Design review of the part built by this model. Coordinates are the model's own, in mm. A direction names the side the tool comes from. Round coordinates to 2 decimals unless told otherwise and drop trailing zeros. Loops run counter-clockwise (first coordinate to the right, second up) from the corner with the lowest first, then second, coordinate; pieces in that order, holes last. Notation, with made-up numbers: (25.5, 57.25) -> (55.5, 57.25) arc R25 ccw to (55.5, 75.25) -> close; hole circle Ø5 at (62, -26). An arc over 180 degrees is marked (long way). Write each question's results on one line, items separated by ' | '. Start each with the question number.
from build123d import *

# Parameters (mm, degrees)
F0_W      = 113
F0_H      = 75
F1_DEPTH  = 0.6
F2_W      = 113
F2_H      = 15
F3_DEPTH  = 1.8
F5_W      = 30
F5_H      = 8
F6_DEPTH  = 39
F8_DEPTH  = 3.4
F10_DEPTH = 4
F12_DEPTH = 2.4
F14_DEPTH = 28
F15_W     = 4
F15_H     = 2
F16_DEPTH = 5.4
F18_DEPTH = 9
F19_R     = 3
F22_DEPTH = 13
F24_DEPTH = 4
F25_R     = 1.6
F26_DEPTH = 2.4
F28_DEPTH = 1
F29_W     = 3
F29_H     = 2.8
F30_DEPTH = 5.6
F31_W     = 6
F31_H     = 3
F32_DEPTH = 3
F33_W     = 6
F33_H     = 3
F34_DEPTH = 6
F35_R     = 2
F36_DEPTH = 4


with BuildPart() as f1:
    # F0 (on Top) → F1 (new body)
    with BuildSketch(Plane.XY):
        with Locations((0, 37.5)):
            Rectangle(F0_W, F0_H)
    extrude(amount=F1_DEPTH)

    # F2 (on face) → F3 (join)
    with BuildSketch(Plane.XY.offset(0.6)):
        with Locations((0, 67.5)):
            Rectangle(F2_W, F2_H)
    extrude(amount=F3_DEPTH)

    # F5 (on offset) → F6 (join)
    with BuildSketch(Plane.YZ.offset(10)):
        with Locations((21, 4.6)):
            Rectangle(F5_W, F5_H)
    extrude(amount=F6_DEPTH)

    # F7 (on face) → F8 (join)
    with BuildSketch(Plane.XY.offset(0.6)):
        Polygon((-26, 17), (-54, 17), (-54, 8), (10, 8), (10, 39), (-26, 39), align=None)
    extrude(amount=F8_DEPTH)

    # F9 (on face) → F10 (join)
    with BuildSketch(Plane.XY.offset(4)):
        Polygon((-26, 26.13884), (-26, 17), (1.574617, 21.862149), (0.011783, 30.725419), align=None)
    extrude(amount=F10_DEPTH)

    # F11 (on face) → F12 (join)
    with BuildSketch(Plane.XY.offset(0.6)):
        with BuildLine():
            Line((-26, 39), (-19, 39))
            Line((-19, 39), (-22.779166, 43.858928))
            ThreePointArc((-22.779166, 43.858928), (-24.784166, 44.456406), (-26, 42.753835))
            Line((-26, 42.753835), (-26, 39))
        make_face()
    extrude(amount=F12_DEPTH)

    # F13 (on face) → F14 (join)
    with BuildSketch(Plane(origin=(-26, 0, 0), x_dir=(0, -1, 0), z_dir=(-1, 0, 0))):
        with BuildLine():
            ThreePointArc((-26.552914, 6.395555), (-30.374719, 4.530004), (-32, 0.6))
            Line((-32, 0.6), (-25, 0.6))
            Line((-25, 0.6), (-26.552914, 6.395555))
        make_face()
    extrude(amount=F14_DEPTH)

    # F15 (on face) → F16 (join)
    with BuildSketch(Plane.XY.offset(0.6)):
        with Locations((-45, 29.4)):
            Rectangle(F15_W, F15_H)
        with Locations((-36, 29.4)):
            Rectangle(F15_W, F15_H)
    extrude(amount=F16_DEPTH)

    # F17 (on face) → F18 (join)
    with BuildSketch(Plane.XY.offset(0.6)):
        with BuildLine():
            Line((18.5, 45.616959), (29.971529, 62))
            ThreePointArc((29.971529, 62), (18.5, 65.616959), (7.028471, 62))
            Line((7.028471, 62), (18.5, 45.616959))
        make_face()
    extrude(amount=F18_DEPTH)

    # F19
    f19_edges = [f1.edges().sort_by_distance(p)[0] for p in [
        (18.5, 45.616959, 5.1),
    ]]
    fillet(f19_edges, radius=F19_R)

    # F21 (on offset) → F22 (join)
    with BuildSketch(Plane.YZ.offset(5)):
        with BuildLine():
            Line((48.073068, 0), (52.926932, 0))
            ThreePointArc((52.926932, 0), (52.981666, 0.297784), (53, 0.6))
            ThreePointArc((53, 0.6), (52.922078, 1.219303), (52.693171, 1.8))
            ThreePointArc((52.693171, 1.8), (49.592442, 2.92945), (48.073068, 0))
        make_face()
        with BuildLine():
            ThreePointArc((52.693171, 1.8), (52.922078, 1.219303), (53, 0.6))
            Line((53, 0.6), (56, 0.6))
            Line((56, 0.6), (56, 1.8))
            Line((56, 1.8), (52.693171, 1.8))
        make_face()
    extrude(amount=-F22_DEPTH)

    # F23 (on face) → F24 (join)
    with BuildSketch(Plane(origin=(-8, 0, 0), x_dir=(0, -1, 0), z_dir=(-1, 0, 0))):
        with BuildLine():
            Line((-52.197056, 0), (-48.802944, 0))
            ThreePointArc((-48.802944, 0), (-50.5, 2.4), (-52.197056, 0))
        make_face()
    extrude(amount=F24_DEPTH)

    # F25 (on face) → F26 (join)
    with BuildSketch(Plane.XY.offset(0.6)):
        with Locations((-15, 56)):
            Circle(F25_R)
    extrude(amount=F26_DEPTH)

    # F27 (on face) → F28 (join)
    with BuildSketch(Plane.XY.offset(0.6)):
        with BuildLine():
            ThreePointArc((-13.612875, 55.202576), (-14.202576, 57.387125), (-16.387125, 56.797424))
            Line((-16.387125, 56.797424), (-20.872636, 48.994848))
            ThreePointArc((-20.872636, 48.994848), (-20.282935, 46.8103), (-18.098387, 47.4))
            Line((-18.098387, 47.4), (-13.612875, 55.202576))
        make_face()
    extrude(amount=F28_DEPTH)

    # F29 (on face) → F30 (join)
    with BuildSketch(Plane.XY.offset(2.4)):
        with Locations((55, 70.6)):
            Rectangle(F29_W, F29_H)
        with Locations((55, 64.6)):
            Rectangle(F29_W, F29_H)
    extrude(amount=F30_DEPTH)

    # F31 (on face) → F32 (cut)
    with BuildSketch(Plane.XY.offset(2.4)):
        with Locations((-53.5, 70.5)):
            Rectangle(F31_W, F31_H)
        with Locations((-53.5, 64.5)):
            Rectangle(F31_W, F31_H)
    extrude(amount=-F32_DEPTH, mode=Mode.SUBTRACT)

    # F33 (on face) → F34 (join)
    with BuildSketch(Plane.XY.offset(0.6)):
        with Locations((53.5, 1.5)):
            Rectangle(F33_W, F33_H)
        with Locations((-38.5, 1.5)):
            Rectangle(F33_W, F33_H)
    extrude(amount=F34_DEPTH)

    # F35 (on face) → F36 (cut)
    with BuildSketch(Plane.XZ):
        with Locations((53.5, 3.6)):
            Circle(F35_R)
        with Locations((-38.5, 3.6)):
            Circle(F35_R)
    extrude(amount=-F36_DEPTH, mode=Mode.SUBTRACT)


solid = f1.part
1) For faces 4 (the face through (51, 3, 4)), 5 (the face through (-54, 63, 1)), 6 (the face through (11.472, 55.653, 5.037)), 7 (the face through (-26, 37, 2)), list the 3-axis set-ups (+Z, -Z, +X, -X, +Y, -Y) from which the entire face can be reached by the end or side of a thin tool; tool diameter is ignored.
2) Take a section at A-A (y = 34). Write out the cut boundary in (x, z), plus the area to 3 significant figures.
3) Take a section at C-C (x = -15). Write out the cut boundary in (y, z).
4) Insertion check: pin 1 (2 mm diameter, centred on y = 51, z = 2, fed in from +X); pin 2 (2.5 mm diameter, centred on y = 25.5, z = 6.5, fed in from +X); pin 3 (1.5 mm diameter, centred on x = -23.5, y = 51.5, fed in from +Z). Each pin has a flat end and moves straight along its axis. Give the tip position at first contact, or say it passes through.
5) To check wall thickness, follow line 1 (Z direction, x = 53.5, y = 1.15); line 2 (Y direction, x = -9, z = 1.75); line 3 (Y direction, x = -15, z = 2.75). State the ranges of each line that lie inside material, in increasing order. Write a range as from..to.
6) Take a section at B-B (x = 3.5). Write out the cut boundary in (y, z).
7) The part is to be moulded in two halves that separate along X. For faces 1 (the face through (-54, 66, 1)), 2 (the face through (-56.5, 73, 1)), 3 (the face through (-39.804, 30.333, 4.574)), say which applies: +X half, -X half, draft (parallel to the pull), parting line (faces both ways), or undercut.
8) Take a section at D-D (y = 50.5). Write out the cut boundary in (x, z), plus the area to 3 significant figures.
Geometry check:
1) face 4: +Z, +X, -X | face 5: +Z, -Z, -X | face 6: +Z | face 7: +Z, -X
2) outline: (-56.5, 0) -> (56.5, 0) -> (56.5, 0.6) -> (49, 0.6) -> (49, 8.6) -> (10, 8.6) -> (10, 4) -> (-26, 4) -> (-26, 0.6) -> (-56.5, 0.6) -> close | area: 502 mm^2
3) outline: (0, 0) -> (75, 0) -> (75, 2.4) -> (60, 2.4) -> (60, 0.6) -> (57.6, 0.6) -> (57.6, 3) -> (54.4, 3) -> (54.4, 1.6) -> (52.79, 1.6) -> (52.79, 0.6) -> (39, 0.6) -> (39, 4) -> (28.08, 4) -> (28.08, 8) -> (18.94, 8) -> (18.94, 4) -> (8, 4) -> (8, 0.6) -> (0, 0.6) -> close
4) pin 1: stops at x = 22.97 | pin 2: stops at x = 49 | pin 3: stops at z = 0.6
5) line 1: z = 0..1.6, 5.6..6.6 | line 2: y = 8..39, 49.12..51.88, 60..75 | line 3: y = 8..39, 54.4..57.6
6) outline: (0, 0) -> (75, 0) -> (75, 2.4) -> (60, 2.4) -> (60, 0.6) -> (56, 0.6) -> (56, 1.8) -> (52.69, 1.8) arc R2.5 ccw to (48, 0.6) -> (39, 0.6) -> (39, 4) -> (8, 4) -> (8, 0.6) -> (0, 0.6) -> close
7) face 1: draft | face 2: -X half | face 3: undercut
8) outline: (-56.5, 0) -> (56.5, 0) -> (56.5, 0.6) -> (21.92, 0.6) -> (21.92, 9.6) -> (15.08, 9.6) -> (15.08, 0.6) -> (5, 0.6) -> (5, 3.1) -> (-8, 3.1) -> (-8, 2.4) -> (-12, 2.4) -> (-12, 0.6) -> (-16.32, 0.6) -> (-16.32, 1.6) -> (-20.01, 1.6) -> (-20.01, 0.6) -> (-56.5, 0.6) -> close | area: 173 mm^2
